from build123d import *

# Parameters (mm, degrees)
F1_DEPTH = 63.5
F0_W     = 19.148961
F0_H     = 19.05
F2_DEPTH = 25.4
F3_DEPTH = 7.9375
F5_R     = 6.35


with BuildPart() as f1:
    # F0 (on Front) → F1 (new body, symmetric)
    with BuildSketch(Plane.XZ):
        Polygon((22.225, 9.525), (-41.275, 9.525), (-41.275, -9.525), (41.275, -9.525), (41.275, 9.525), align=None)
    extrude(amount=F1_DEPTH, both=True)

    # F0 (on Front) → F2 (join, symmetric)
    with BuildSketch(Plane.XZ):
        with Locations((69.89948, 52.38242)):
            Rectangle(F0_W, F0_H)
        with BuildLine():
            Line((22.225, 26.98242), (22.225, 9.525))
            Line((22.225, 9.525), (41.275, 9.525))
            Line((41.275, 9.525), (41.275, 26.98242))
            ThreePointArc((41.275, 26.98242), (45.92468, 38.20774), (57.15, 42.85742))
            Line((57.15, 42.85742), (60.325, 42.85742))
            Line((60.325, 42.85742), (60.325, 61.90742))
            Line((60.325, 61.90742), (57.15, 61.90742))
            ThreePointArc((57.15, 61.90742), (32.454296, 51.678124), (22.225, 26.98242))
        make_face()
    extrude(amount=F2_DEPTH, both=True)

    # F0 (on Front) → F3 (join, symmetric)
    with BuildSketch(Plane.XZ):
        with BuildLine():
            add(Edge.make_bspline(
                [(-41.275, 9.525), (-30.242277, 40.943753), (28.724005, 65.23551), (57.15, 61.90742)],
                knots=[0, 0, 0, 0, 111.496182, 111.496182, 111.496182, 111.496182], degree=3))
            Line((-41.275, 9.525), (22.225, 9.525))
            Line((22.225, 9.525), (22.225, 26.98242))
            ThreePointArc((22.225, 26.98242), (32.454296, 51.678124), (57.15, 61.90742))
        make_face()
    extrude(amount=F3_DEPTH, both=True)

    # F0 (on Front) → F4 (revolve)
    with BuildSketch(Plane.XZ):
        Polygon((79.473961, 66.675), (79.473961, 61.90742), (79.473961, 42.85742), (79.473961, 38.1), (111.125, 38.1), (111.125, 66.675), align=None)
    revolve(axis=Axis((79.473961, 0, 52.38242), (0, 0, -1)))

    # F5
    f5_edges = [f1.edges().sort_by_distance(p)[0] for p in [
        (-41.275, -63.5, 0),
        (41.275, -63.5, 0),
        (-41.275, 63.5, 0),
        (41.275, 63.5, 0),
    ]]
    fillet(f5_edges, radius=F5_R)


solid = f1.part
Here's how the part is built. I have some questions about the finished solid (model axes, mm). A direction names the side the tool comes from. Give positions to 0.01 mm unless a question says otherwise; leave off trailing zeros. Loops run counter-clockwise (first coordinate to the right, second up) from the corner with the lowest first, then second, coordinate; pieces in that order, holes last. Notation, with made-up numbers: (72, 86.5) -> (85, 86.5) arc R23 ccw to (85, 114.5) -> close; hole circle Ø4 at (19.25, -7.75). An arc over 180 degrees is marked (long way). Answer as a JSON object with one key per item and string values. Group by question number.
Item 1: Imagine slicing it at A-A on y = -44. Write out the boundary of the cut face in (x, z) (3 decimals), then the cut area to 3 significant figures.
Item 2: On a 3-axis mill with a long thin cutter (end or side, diameter ignored), from which of +Z, -Z, +X, -X, +Y, -Y can I reach the whole of each face in a straight line? I mean faces 1 (the flat face through (4, 7.938, 30)), 2 (the flat face through (4, -7.938, 30)), 3 (the flat face through (41.275, -1, 4)). Say none if no direction works.
Item 3: Thinking about a two-plate mould opening in X: for faces 4 (the flat face through (80, 0, 38.1)), 5 (the flat face through (22.225, 17, 18)), 6 (the cylindrical face through (44.047, -0.356, 35.944)), 7 (the cylindrical face through (39.464, 61.59, 0.133)), which applies, pulls with the +X half, pulls with the -X half, needs draft (parallel to the pull), parting line crosses it, or undercut?
Item 4: I need wall thicknesses on L1, parallel to Y at x = 30, z = 33; L2, parallel to X at y = 27, z = 7 (3 decimals); L3, parallel to Z at x = 9, y = 49.5 (3 decimals). Which ranges of each line are inside material? Lowest first, please.
Item 5: Imagine slicing it at B-B on x = 51. Write out the boundary of the cut face in (y, z) (3 decimals).
Item 6: Will these pins go through, and if not, where does the flat tip stop? pin 1 (16 mm diameter, centred on x = 25, z = 37.5, fed in from -Y); pin 2 (6 mm diameter, centred on y = -21.5, z = 56.5, fed in from +X); pin 3 (14 mm diameter, centred on y = -21, z = 20.5, fed in from -X) (3 decimals); pin 4 (10 mm diameter, centred on x = 46.5, z = 21, fed in from -Y).
Answer list:
{
 "1": {"outline": "(-41.275, -9.525) -> (41.275, -9.525) -> (41.275, 9.525) -> (-41.275, 9.525) -> close", "area": "1,570 mm2"},
 "2": {"face 1": "+Z, -X, +Y", "face 2": "+Z, -X, -Y", "face 3": "-Z, +X, +Y, -Y"},
 "3": {"face 4": "needs draft", "face 5": "pulls with the -X half", "face 6": "undercut", "face 7": "pulls with the +X half"},
 "4": {"L1": "y = -25.4 to 25.4", "L2": "x = -41.275 to 41.275", "L3": "z = -9.525 to 9.525"},
 "5": {"outline": "(-25.4, 41.618) -> (-13.821, 41.618) -> (-13.821, 38.1) -> (13.821, 38.1) -> (13.821, 41.618) -> (25.4, 41.618) -> (25.4, 61.362) -> (13.821, 61.362) -> (13.821, 66.675) -> (-13.821, 66.675) -> (-13.821, 61.362) -> (-25.4, 61.362) -> close"},
 "6": {"pin 1": "stops at y = -25.4", "pin 2": "stops at x = 105.16", "pin 3": "stops at x = 22.225", "pin 4": "passes through"}
}
